The model under review builds one solid part; all positions refer to its coordinate system, in mm. Face numbers are marked on the shaded views. A direction names the side the tool comes from. Round coordinates to 2 decimals unless told otherwise and drop trailing zeros. Loops run counter-clockwise (first coordinate to the right, second up) from the corner with the lowest first, then second, coordinate; pieces in that order, holes last. Notation, with made-up numbers: (12, -23.75) -> (66, -23.75) arc R23 ccw to (66, -1.75) -> close; hole circle Ø2 at (-32.75, -12). An arc over 180 degrees is marked (long way). Write each question's results on one line, items separated by ' | '. Start each with the question number.
Item 1: We need section A-A (y = 34.5). Give the boundary of the cut face in (x, z), and give its area (3 significant figures).
Item 2: We need section D-D (y = 116.5). Give the boundary of the cut face in (x, z), and give its area (3 significant figures).
Item 3: Clearance check with flat-ended pins moving along their axes: pin 1 Ø5 at (x, y) = (94, 21.5) entering from +Z; pin 2 Ø1 at (x, y) = (-56.5, 98) entering from -Z; pin 3 Ø12.5 at (y, z) = (80, 69.5) entering from -X. State where each tip first meets the part, or that it passes through.
Item 4: We need section C-C (x = 88). Give the boundary of the cut face in (y, z), and give its area (3 significant figures).
Item 5: We need section B-B (z = 6.5). Give the boundary of the cut face in (x, y), and give its area (3 significant figures).
Item 6: Tool access review of the marked faces 1, 2, 3, 4 and 5: name each direction out of +Z, -Z, +X, -X, +Y, -Y from which nothing blocks a thin tool from reaching the whole face with its end or side.
Item 7: For L1, parallel to Z at x = 70.5, y = 15; L2, parallel to X at y = 102.5, z = 68.5; L3, parallel to X at y = 59, z = -55, list the stretches that pass through material, from the lowest coordinate up. Write a range as from..to.
from build123d import *

# Parameters (mm, degrees)
SKETCH1_W           = 64.856187625
SKETCH1_H           = 53.867265469
SKETCH1_W_2         = 50.216999898
SKETCH1_H_2         = 56.395605674
BOSS_EXTRUDE1_DEPTH = 144.78
CHAMFER1_SIZE       = 65.88
CHAMFER1_SIZE2      = 73.167152477
CHAMFER2_SIZE       = 27.78
CHAMFER2_SIZE2      = 39.673951627


with BuildPart() as part:
    # Sketch1 → Boss-Extrude1 (new body)
    with BuildSketch(Plane(origin=(0, 0, 0), x_dir=(1, 0, 0), z_dir=(0, 1, 0))):
        with Locations((-59.723790396, -26.933632735)):
            Rectangle(SKETCH1_W, SKETCH1_H)
        with Locations((-59.723790396, 26.933632735)):
            Rectangle(SKETCH1_W, SKETCH1_H)
        Polygon((-27.295696583, 53.867265469), (-27.295696583, 0), (67.459562421, 0), (67.459562421, 56.395605674), (67.459562421, 95.440559589), (-27.295696583, 95.440559589), align=None)
        Polygon((67.459562421, 0), (-27.295696583, 0), (-27.295696583, -53.867265469), (-27.295696583, -95.440559589), (67.459562421, -95.440559589), (67.459562421, -56.395605674), align=None)
        with Locations((92.56806237, 28.197802837)):
            Rectangle(SKETCH1_W_2, SKETCH1_H_2)
        with Locations((92.56806237, -28.197802837)):
            Rectangle(SKETCH1_W_2, SKETCH1_H_2)
    extrude(amount=BOSS_EXTRUDE1_DEPTH)

    # Chamfer1
    chamfer1_edges = [part.edges().sort_by_distance(p)[0] for p in [
        (-92.151884208, 144.78, 0),
    ]]
    chamfer1_side = [part.faces().sort_by_distance(p)[0] for p in [
        (15.2977171, 144.78, 0),
    ]]
    chamfer(chamfer1_edges, length=CHAMFER1_SIZE, length2=CHAMFER1_SIZE2, reference=chamfer1_side[0])

    # Chamfer2
    chamfer2_edges = [part.edges().sort_by_distance(p)[0] for p in [
        (-27.295696583, 71.821470582, -95.440559589),
    ]]
    chamfer2_side = [part.faces().sort_by_distance(p)[0] for p in [
        (20.083928703, 72.386944526, -95.440559589),
    ]]
    chamfer(chamfer2_edges, length=CHAMFER2_SIZE, length2=CHAMFER2_SIZE2, reference=chamfer2_side[0])


solid = part.part
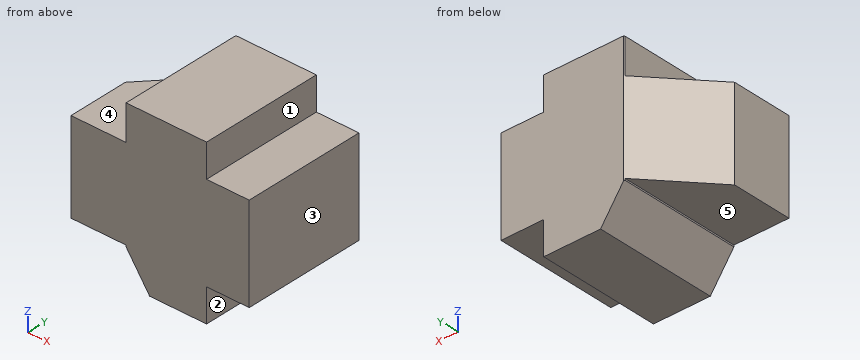
Here are the results:
1) outline: (-92.15, -53.87) -> (-27.3, -53.87) -> (-27.3, -55.77) -> (0.48, -95.44) -> (67.46, -95.44) -> (67.46, -56.4) -> (117.68, -56.4) -> (117.68, 56.4) -> (67.46, 56.4) -> (67.46, 95.44) -> (-27.3, 95.44) -> (-27.3, 53.87) -> (-92.15, 53.87) -> close | area: 30,200 mm2
2) outline: (-51.74, -53.87) -> (-27.3, -53.87) -> (-27.3, -55.77) -> (0.48, -95.44) -> (67.46, -95.44) -> (67.46, -56.4) -> (117.68, -56.4) -> (117.68, 56.4) -> (67.46, 56.4) -> (67.46, 95.44) -> (-27.3, 95.44) -> (-27.3, 53.87) -> (-51.74, 53.87) -> close | area: 25,800 mm2
3) pin 1: stops at z = 56.4 | pin 2: stops at z = -53.87 | pin 3: stops at x = -27.3
4) outline: (0, -56.4) -> (144.78, -56.4) -> (144.78, 56.4) -> (0, 56.4) -> close | area: 16,300 mm2
5) outline: (-92.15, 0) -> (117.68, 0) -> (117.68, 144.78) -> (-26.27, 144.78) -> (-92.15, 71.61) -> close | area: 28,000 mm2
6) face 1: +Z, +X, +Y, -Y | face 2: -Z, +X, +Y, -Y | face 3: +Z, -Z, +X, +Y, -Y | face 4: +Z, -X, +Y, -Y | face 5: -Z, -X, +Y, -Y
7) L1: z = -56.4..56.4 | L2: x = -27.3..67.46 | L3: x = -27.3..117.68
